from build123d import *

# Parameters (mm, degrees)
MODEL_W             = 1.574799418
MODEL_H             = 12.699998915
BOSS_EXTRUDE1_DEPTH = 3.048


with BuildPart() as part:
    # Model → Boss-Extrude1 (new body)
    with BuildSketch(Plane.XY):
        with BuildLine():
            Line((15.63479994, 91.058996506), (5.17, 91.058996506))
            Line((5.17, 91.058996506), (5.17, 97.154987045))
            Line((5.17, 97.154987045), (30.823999648, 97.154987045))
            Line((30.823999648, 97.154987045), (30.823999648, 67.817998119))
            Line((30.823999648, 67.817998119), (27.648999919, 67.817998119))
            Line((27.648999919, 67.817998119), (27.648999919, 56.261000223))
            Line((27.648999919, 56.261000223), (30.823999648, 56.261000223))
            Line((30.823999648, 56.261000223), (30.823999648, 9.397999849))
            Line((30.823999648, 9.397999849), (27.648999919, 9.397999849))
            Line((27.648999919, 9.397999849), (27.648999919, 0))
            Line((27.648999919, 0), (19.724199181, 0))
            Line((19.724199181, 0), (19.724199181, 3.047999926))
            Line((19.724199181, 3.047999926), (13.424999644, 3.047999926))
            Line((13.424999644, 3.047999926), (13.424999644, 0))
            Line((13.424999644, 0), (5.17, 0))
            Line((5.17, 0), (5.17, 9.397999849))
            Line((5.17, 9.397999849), (5.17, 9.51))
            Line((5.17, 9.51), (2.5, 9.51))
            Line((2.5, 9.51), (0, 12.01))
            Line((0, 12.01), (0, 37.8165))
            ThreePointArc((0, 37.8165), (0.439339828, 38.877160172), (1.5, 39.3165))
            Line((1.5, 39.3165), (5.17, 39.3165))
            Line((5.17, 39.3165), (5.17, 51.9965))
            Line((5.17, 51.9965), (1.5, 51.9965))
            ThreePointArc((1.5, 51.9965), (0.439339828, 52.435839828), (0, 53.4965))
            Line((0, 53.4965), (0, 79.303))
            Line((0, 79.303), (2.5, 81.803))
            Line((2.5, 81.803), (5.17, 81.803))
            Line((5.17, 81.803), (5.17, 88.011001237))
            Line((5.17, 88.011001237), (15.63479994, 88.011001237))
            Line((15.63479994, 88.011001237), (15.63479994, 91.058996506))
        make_face()
        with Locations((27.166399737, 81.661001779)):
            Rectangle(MODEL_W, MODEL_H, mode=Mode.SUBTRACT)
    extrude(amount=BOSS_EXTRUDE1_DEPTH)


solid = part.part
The listing builds one solid part. Answer for the finished solid, in the listing's coordinates (mm). A direction names the side the tool comes from. Round coordinates to 2 decimals unless told otherwise and drop trailing zeros. Write each loop counter-clockwise with the first axis right and the second up, starting at its lowest first coordinate (ties: lowest second). Pieces come first, ordered by that corner, then holes. Notation, with made-up numbers: M -22,74 L 14,74 A19 ccw 14,93 Z; hole C 4,51.25 d10. An arc over 180 degrees is marked long. Write each question's results on one line, items separated by ' | '. Start each with the question number.
Item 1: Straight lines are drawn through the part: probe 1 along X at (y, z) = (61, 2.85); probe 2 along Y at (x, z) = (19, 0.9); probe 3 along X at (y, z) = (41.5, 1). For each, find the intervals that lie inside material, in ascending order.
Item 2: Given pin 1 Ø0.9 at (x, z) = (29, 1) entering from -Y; pin 2 Ø1 at (x, z) = (4, 2) entering from -Y; pin 3 Ø0.9 at (y, z) = (2.5, 1) entering from +X, each flat-ended and moving along its own axis, determine where each tip first touches the part or whether it passes through.
Item 3: Find section C-C on x = 7. Write down the section's boundary in (y, z).
Item 4: Which of the six approach directions +Z, -Z, +X, -X, +Y, -Y give full straight-line access (tool end or side, diameter ignored) to faces 4 (the flat face through (5.17, 94, 2)), 5 (the flat face through (27.649, 5, 2)), 6 (the flat face through (27.649, 62, 2)), 7 (the flat face through (10, 91.059, 2)), 8 (the flat face through (27, 75.311, 2))?
Item 5: Find section D-D on x = 16.5. Write down the section's boundary in (y, z), and give its area (3 significant figures).
Item 6: The mould has two halves that part along X. Classify faces 1 (the flat face through (17, 3.048, 2)), 2 (the flat face through (29, 9.398, 2)), 3 (the flat face through (5.17, 5, 2)): +X half, -X half, draft (parallel to the pull), parting line (faces both ways), or undercut.
Item 7: Find section A-A on y = 78. Write down the section's boundary in (x, z).
Answer block:
1) probe 1: x = 0 to 27.65 | probe 2: y = 3.05 to 97.15 | probe 3: x = 5.17 to 30.82
2) pin 1: stops at y = 9.4 | pin 2: stops at y = 9.51 | pin 3: stops at x = 27.65
3) outline: M 0,0 L 88.01,0 L 88.01,3.05 L 0,3.05 Z; M 91.06,0 L 97.15,0 L 97.15,3.05 L 91.06,3.05 Z
4) face 4: +Z, -Z, -X, +Y | face 5: +Z, -Z, +X, -Y | face 6: +Z, -Z, +X | face 7: +Z, -Z, -X | face 8: +Z, -Z
5) outline: M 3.05,0 L 97.15,0 L 97.15,3.05 L 3.05,3.05 Z | area: 287 mm²
6) face 1: undercut | face 2: draft | face 3: -X half
7) outline: M 0,0 L 26.38,0 L 26.38,3.05 L 0,3.05 Z; M 27.95,0 L 30.82,0 L 30.82,3.05 L 27.95,3.05 Z
